For this review, take the finished solid that the model builds, in its own axes (mm). Round coordinates to 2 decimals unless told otherwise and drop trailing zeros. Loops run counter-clockwise (first coordinate to the right, second up) from the corner with the lowest first, then second, coordinate; pieces in that order, holes last. Notation, with made-up numbers: (-38.75, 63.25) -> (19.25, 63.25) arc R21 cw to (19.25, 91.25) -> close; hole circle Ø6 at (13.25, 10.5). An arc over 180 degrees is marked (long way). Use one line per item in the form item = value. Start each with the question number.
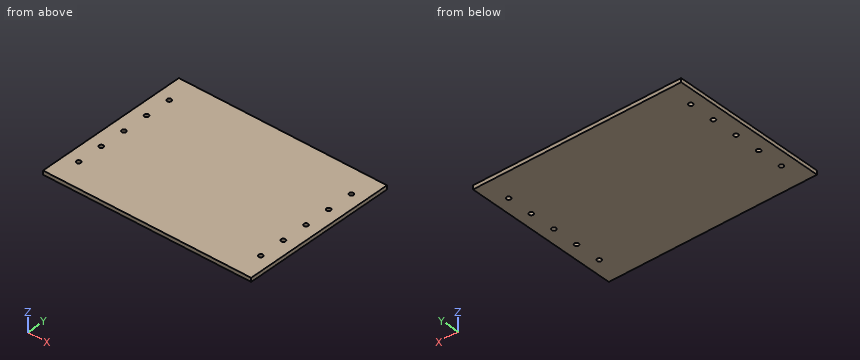
from build123d import *

# Parameters (mm, degrees)
SKETCH_1_W      = 160
SKETCH_1_H      = 120
SKETCH_1_R      = 1.65
EXTRUDE_1_DEPTH = 3


with BuildPart() as part:
    # 草图1 → 凸台-拉伸1 (new body)
    with BuildSketch(Plane.XY):
        Rectangle(SKETCH_1_W, SKETCH_1_H)
        with Locations((-70, 40)):
            Circle(SKETCH_1_R, mode=Mode.SUBTRACT)
        with Locations((-70, 20)):
            Circle(SKETCH_1_R, mode=Mode.SUBTRACT)
        with Locations((-70, 0)):
            Circle(SKETCH_1_R, mode=Mode.SUBTRACT)
        with Locations((-70, -20)):
            Circle(SKETCH_1_R, mode=Mode.SUBTRACT)
        with Locations((-70, -40)):
            Circle(SKETCH_1_R, mode=Mode.SUBTRACT)
        with Locations(Location((70, -40, 0), (0, 0, 180))):
            Circle(SKETCH_1_R, mode=Mode.SUBTRACT)
        with Locations(Location((70, -20, 0), (0, 0, 180))):
            Circle(SKETCH_1_R, mode=Mode.SUBTRACT)
        with Locations(Location((70, 0, 0), (0, 0, 180))):
            Circle(SKETCH_1_R, mode=Mode.SUBTRACT)
        with Locations(Location((70, 20, 0), (0, 0, 180))):
            Circle(SKETCH_1_R, mode=Mode.SUBTRACT)
        with Locations(Location((70, 40, 0), (0, 0, 180))):
            Circle(SKETCH_1_R, mode=Mode.SUBTRACT)
    extrude(amount=EXTRUDE_1_DEPTH)


solid = part.part
Item 1: For P1, Ø2.5, axis at x = -70, y = 20, coming from the +Z side, flat-tipped, find the tip position at first contact; note if it passes through.
Item 2: Take a section at B-B on x = 70. Give the boundary of the cut face in (y, z), plus the area to 4 significant figures.
Item 3: Take a section at A-A on y = 0. Give the boundary of the cut face in (x, z), plus the area to 3 significant figures.
Item 4: Wall thickness on line 1 (Y direction, x = -70, z = 1.65); line 2 (X direction, y = 38.5, z = 1.4): over which ranges is each line inside the solid? List them lowest first.
Results:
q1.P1 = through
q2.outline = (-60, 0) -> (-41.65, 0) -> (-41.65, 3) -> (-60, 3) -> close; (-38.35, 0) -> (-21.65, 0) -> (-21.65, 3) -> (-38.35, 3) -> close; (-18.35, 0) -> (-1.65, 0) -> (-1.65, 3) -> (-18.35, 3) -> close; (1.65, 0) -> (18.35, 0) -> (18.35, 3) -> (1.65, 3) -> close; (21.65, 0) -> (38.35, 0) -> (38.35, 3) -> (21.65, 3) -> close; (41.65, 0) -> (60, 0) -> (60, 3) -> (41.65, 3) -> close
q2.area = 310.5 mm2
q3.outline = (-80, 0) -> (-71.65, 0) -> (-71.65, 3) -> (-80, 3) -> close; (-68.35, 0) -> (68.35, 0) -> (68.35, 3) -> (-68.35, 3) -> close; (71.65, 0) -> (80, 0) -> (80, 3) -> (71.65, 3) -> close
q3.area = 460 mm2
q4.line_1 = -60 to -41.65, -38.35 to -21.65, -18.35 to -1.65, 1.65 to 18.35, 21.65 to 38.35, 41.65 to 60
q4.line_2 = -80 to -70.69, -69.31 to 69.31, 70.69 to 80
